from build123d import *

# Parameters (mm, degrees)
F0_W     = 304.8
F0_H     = 76.2
F1_DEPTH = 6.35
F3_DEPTH = 76.2
F5_W     = 304.7997951508
F5_H     = 76.2000009418
F6_DEPTH = 6.35


with BuildPart() as f1:
    # F0 (on Right) → F1 (new body)
    with BuildSketch(Plane.YZ):
        with Locations((152.4, 38.1)):
            Rectangle(F0_W, F0_H)
    extrude(amount=F1_DEPTH)

    # F2 (on Right) → F3 (join)
    with BuildSketch(Plane.YZ):
        Polygon((304.7999739647, 0), (304.7999739647, 76.2000977993), (298.4695136547, 76.2183889747), (298.4695136547, 0), align=None)
    extrude(amount=F3_DEPTH)

    # F5 (on offset) → F6 (join)
    with BuildSketch(Plane.YZ.offset(76.2)):
        with Locations((152.3998975754, 38.1000004709)):
            Rectangle(F5_W, F5_H)
    extrude(amount=-F6_DEPTH)


solid = f1.part
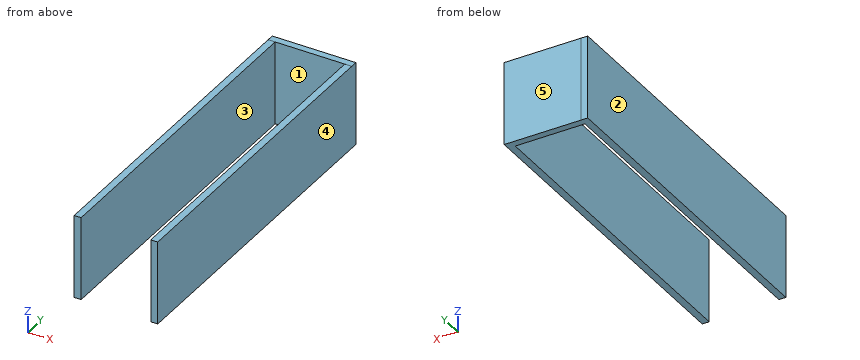
For this review, take the finished solid that the model builds, in its own axes (mm). Face numbers are marked on the shaded views. A direction names the side the tool comes from. Coordinates: 2 decimals unless noted, no trailing zeros. Order: outer loops, then holes, each group sorted by start corner. A loop starts at its lowest first (then second) coordinate and runs counter-clockwise, first axis right, second up. Notation, with made-up numbers: (1, 33) - (12, 33) arc R20 cw to (12, 57) - close; hole circle Ø8 at (80.25, 72.5). An arc over 180 degrees is marked (long way). Answer as CSV lines item,"result". Start each with the question number.
1) Machinability: for the marked faces 1 and 2, which of the approach directions +Z, -Z, +X, -X, +Y, -Y give a long, thin tool a straight path to every point of the face, cutting with its end or side? Answer none if there is none.
2) Insertion check: P1, Ø5, axis at x = 21, z = 20, coming from the -Y side; P2, Ø3, axis at x = 74.5, y = 193.5, coming from the +Z side. Each pin has a flat end and moves straight along its axis. Give the tip position at first contact, or say it passes through.
3) Draft analysis for pull direction X (two halves, no side actions). For the marked faces 3, 4 and 5, state which applies: +X half, -X half, draft (parallel to the pull), parting line (faces both ways), or undercut.
4) Add section A-A (y = 272.5). State the section outline as (x, z) points, then the cut area to 3 significant figures.
5) Add section C-C (x = 20). State the section outline as (y, z) points, then the cut area to 3 significant figures.
6) To check wall thickness, follow line 1 along X through (y, z) = (139.5, 9.5); line 2 along Y through (x, z) = (48, 26); line 3 along Z through (x, y) = (3, 122). State the ranges of each line that lie inside material, in increasing order. Write a range as [from, to].
Result:
1,face 1,"+Z, -Z, -Y"
1,face 2,"+Z, -Z, -X, +Y, -Y"
2,P1,"y = 298.47"
2,P2,"z = 76.2"
3,face 3,"undercut"
3,face 4,"+X half"
3,face 5,"draft"
4,outline,"(0, 0) - (6.35, 0) - (6.35, 76.2) - (0, 76.2) - close; (69.85, 0) - (76.2, 0) - (76.2, 76.2) - (69.85, 76.2) - close"
4,area,"968 mm^2"
5,outline,"(298.47, 0) - (304.8, 0) - (304.8, 76.2) - (298.47, 76.22) - close"
5,area,"482 mm^2"
6,line 1,"[0, 6.35], [69.85, 76.2]"
6,line 2,"[298.47, 304.8]"
6,line 3,"[0, 76.2]"
